from build123d import *

# Parameters (mm, degrees)
F0_W     = 50
F0_H     = 30
F1_DEPTH = 109
F2_R     = 8
F3_DEPTH = 30.001
F4_R     = 5
F5_DEPTH = 50
F6_W     = 30
F6_H     = 20
F7_DEPTH = 109.001
F8_W     = 20
F8_H     = 20
F9_DEPTH = 25


with BuildPart() as f1:
    # F0 (on Front) → F1 (new body)
    with BuildSketch(Plane.XZ):
        with Locations((25, 15)):
            Rectangle(F0_W, F0_H)
    extrude(amount=F1_DEPTH)

    # F2 (on face) → F3 (cut, through all)
    with BuildSketch(Plane.XY.offset(30)):
        with Locations((25, -20)):
            Circle(F2_R)
    extrude(amount=-F3_DEPTH, mode=Mode.SUBTRACT)

    # F4 (on face) → F5 (join)
    with BuildSketch(Plane.YZ.offset(50)):
        Polygon((-52, 0), (-72, 0), (-72, -16), (-68, -20), (-56, -20), (-52, -16), align=None)
        with Locations((-62, -12)):
            Circle(F4_R, mode=Mode.SUBTRACT)
        Polygon((-82, 0), (-102, 0), (-102, -16), (-98, -20), (-86, -20), (-82, -16), align=None)
        with Locations((-92, -12)):
            Circle(F4_R, mode=Mode.SUBTRACT)
    extrude(amount=-F5_DEPTH)

    # F6 (on face) → F7 (cut, through all)
    with BuildSketch(Plane(origin=(0, 0, 0), x_dir=(-1, 0, 0), z_dir=(0, 1, 0))):
        with Locations((-25, -10)):
            Rectangle(F6_W, F6_H)
    extrude(amount=-F7_DEPTH, mode=Mode.SUBTRACT)

    # F8 (on face) → F9 (cut)
    with BuildSketch(Plane.YZ.offset(50)):
        with Locations((-92, -10)):
            Rectangle(F8_W, F8_H)
    extrude(amount=-F9_DEPTH, mode=Mode.SUBTRACT)


solid = f1.part
Build history of the part. All positions in model axes, mm. A direction names the side the tool comes from. Give positions to 0.01 mm unless a question says otherwise; leave off trailing zeros. Order: outer loops, then holes, each group sorted by start corner. A loop starts at its lowest first (then second) coordinate and runs counter-clockwise, first axis right, second up. Notation, with made-up numbers: M 8.5,88 L 27.5,88 A10 ccw 27.5,98 Z; hole C -11,-8 d6. An arc over 180 degrees is marked long. Use one line per item in the form item = value.
Q1. Slice it at B-B, the plane y = -62. Write the cut outline in (x, z), and give its area (3 significant figures).
Conclusion:
outline = M 0,-20 L 10,-20 L 10,-17 L 0,-17 Z; M 0,-7 L 10,-7 L 10,0 L 40,0 L 40,-7 L 50,-7 L 50,30 L 0,30 Z; M 40,-20 L 50,-20 L 50,-17 L 40,-17 Z
area = 1,700 mm2
Q2. Pin check, flat tips, straight feed: P1, Ø16, axis at y = -89.5, z = -14, coming from the +X side; P2, Ø8, axis at x = 7.5, z = -5, coming from the -Y side; P3, Ø8, axis at x = 3, z = -7, coming from the +Y side. Stop position of each tip, or through.
Conclusion:
P1 = 10
P2 = -102
P3 = -52
Q3. Slice it at D-D, the plane x = 20. Write the cut outline in (y, z) (3 decimals), and give its area (3 significant figures).
Conclusion:
outline = M -109,0 L -26.245,0 L -26.245,30 L -109,30 Z; M -13.755,0 L 0,0 L 0,30 L -13.755,30 Z
area = 2,900 mm2
Q4. Which spindle directions (+Z, -Z, +X, -X, +Y, -Y) get a long thin tool onto all of the face, cutting with end or side? Do faces 4 (the flat face through (5, -52, -8)), 5 (the flat face through (5, -82, -8)), 6 (the flat face through (40, -62, -6)). Say none if no direction does.
Conclusion:
face_4 = -Z, +X, -X, +Y
face_5 = -Z, +X, -X
face_6 = -Z, +Y, -Y
Q5. Pull direction Z, two halves, no side cores. Call faces 1 (the flat face through (25, 0, 15)), 2 (the flat face through (45, -70, -18)), 3 (the cylindrical face through (5, -67, -12)): released by +Z, released by -Z, zero draft, split by the parting line, or undercut.
Conclusion:
face_1 = zero draft
face_2 = released by -Z
face_3 = undercut
Q6. Slice it at C-C, the plane z = 27. Write the cut outline in (x, y), and give its area (3 significant figures).
Conclusion:
outline = M 0,-109 L 50,-109 L 50,0 L 0,0 Z; hole C 25,-20 d16
area = 5,250 mm2
Q7. Slice it at A-A, the plane y = -20. Write the cut outline in (x, z).
Conclusion:
outline = M 0,0 L 17,0 L 17,30 L 0,30 Z; M 33,0 L 50,0 L 50,30 L 33,30 Z
Q8. Wall check: probe 1 along Z at (x, y) = (7.5, -62); probe 2 along Z at (x, y) = (32, -89.5); probe 3 along X at (y, z) = (-61.5, -1). Give the ranges that are in metal, low to high.
Conclusion:
probe_1 = -20 to -17, -7 to 30
probe_2 = 0 to 30
probe_3 = 0 to 10, 40 to 50
